Source: CAD feature listing. Evaluate the final solid. Frame: model axes, mm. Give positions to 0.01 mm unless a question says otherwise; leave off trailing zeros. Write each loop counter-clockwise with the first axis right and the second up, starting at its lowest first coordinate (ties: lowest second). Pieces come first, ordered by that corner, then holes. Notation, with made-up numbers: (-40, 45.25) -> (-11, 45.25) arc R24 cw to (-11, 57.25) -> close; hole circle Ø4 at (-27, 60). An arc over 180 degrees is marked (long way). Use one line per item in the form item = value. Start each with the question number.
(1) Cut plane A-A, the plane y = -89. Output: boundary loops of the cut face in (x, z), and give its area (3 significant figures).
(2) Cut plane B-B, the plane x = 65. Output: boundary loops of the cut face in (y, z).
(3) Cut plane C-C, the plane x = 9.5. Output: boundary loops of the cut face in (y, z), and give its area (3 significant figures).
(4) First-contact query: P1, Ø1.5, axis at x = 27.5, z = -1, coming from the -Y side; P2, Ø3, axis at y = -82, z = -4.5, coming from the -X side; P3, Ø1.5, axis at y = -70, z = -2, coming from the -X side; P4, Ø1.5, axis at x = 114, y = -58.5, coming from the +Z side. Flat tips, straight axial feed; report the tip coordinate or a pass-through.
(5) Cut plane D-D, the plane z = -0.85. Count the separate pieces of the cut face and the enclosed holes in it, and give its area (3 significant figures).
(6) Material intervals for line 1 along X through (y, z) = (-136.5, -1.9); line 2 along X through (y, z) = (-113, -2.2); line 3 along X through (y, z) = (-83, -1.7), sorted ascending. Write a range as from..to.
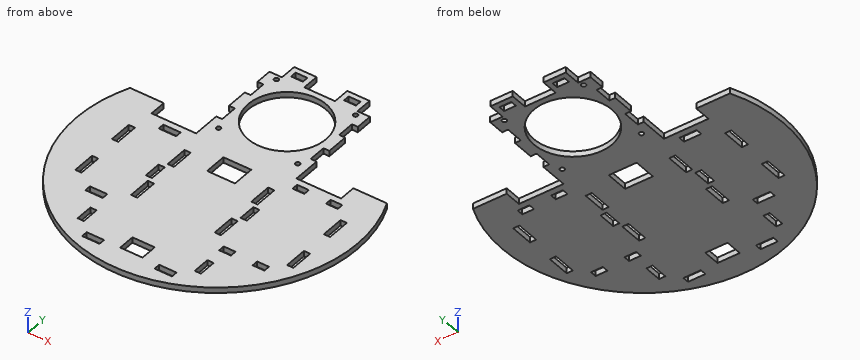
from build123d import *

# Parameters (mm, degrees)
SKETCH1_R           = 35
SKETCH1_R_2         = 2
SKETCH1_W           = 20
SKETCH1_H           = 15
SKETCH1_W_2         = 25
SKETCH1_H_2         = 20
SKETCH1_W_3         = 10.6
SKETCH1_H_3         = 5.6
SKETCH1_W_4         = 15.6
SKETCH1_W_5         = 5.6
SKETCH1_H_4         = 20.6
SKETCH1_H_5         = 15.6
BOSS_EXTRUDE1_DEPTH = 5


with BuildPart() as part:
    # Sketch1 → Boss-Extrude1 (new body)
    with BuildSketch(Plane(origin=(0, 0, 0), x_dir=(-1, 0, 0), z_dir=(0, 0, -1))):
        with BuildLine():
            Line((-25.476672243, 28.966950724), (-36.676672243, 28.966950724))
            Line((-36.676672243, 28.966950724), (-36.676672243, 43.966950724))
            Line((-36.676672243, 43.966950724), (-56.676672243, 43.966950724))
            Line((-56.676672243, 43.966950724), (-56.676672243, 28.966950724))
            Line((-56.676672243, 28.966950724), (-84.276672243, 28.966950724))
            Line((-84.276672243, 28.966950724), (-84.276672243, 43.966950724))
            Line((-84.276672243, 43.966950724), (-104.276672243, 43.966950724))
            Line((-104.276672243, 43.966950724), (-104.276672243, 28.966950724))
            Line((-104.276672243, 28.966950724), (-115.476672243, 28.966950724))
            Line((-115.476672243, 28.966950724), (-115.476672243, 14.266950724))
            Line((-115.476672243, 14.266950724), (-110.176672243, 14.266950724))
            Line((-110.176672243, 14.266950724), (-110.176672243, -1.333049276))
            Line((-110.176672243, -1.333049276), (-115.476672243, -1.333049276))
            Line((-115.476672243, -1.333049276), (-115.476672243, -20.733049276))
            Line((-115.476672243, -20.733049276), (-110.176672243, -20.733049276))
            Line((-110.176672243, -20.733049276), (-110.176672243, -36.333049276))
            Line((-110.176672243, -36.333049276), (-115.476672243, -36.333049276))
            Line((-115.476672243, -36.333049276), (-115.476672243, -61.033049276))
            Line((-115.476672243, -61.033049276), (-155.476672243, -61.033049276))
            Line((-155.476672243, -61.033049276), (-155.476672243, -46.033049276))
            Line((-155.476672243, -46.033049276), (-185.693858461, -46.033049276))
            ThreePointArc((-185.693858461, -46.033049276), (-70.476672243, -223.033049276), (44.740513975, -46.033049276))
            Line((44.740513975, -46.033049276), (14.523327757, -46.033049276))
            Line((14.523327757, -46.033049276), (14.523327757, -61.033049276))
            Line((14.523327757, -61.033049276), (-25.476672243, -61.033049276))
            Line((-25.476672243, -61.033049276), (-25.476672243, -36.333049276))
            Line((-25.476672243, -36.333049276), (-30.776672243, -36.333049276))
            Line((-30.776672243, -36.333049276), (-30.776672243, -20.733049276))
            Line((-30.776672243, -20.733049276), (-25.476672243, -20.733049276))
            Line((-25.476672243, -20.733049276), (-25.476672243, -1.333049276))
            Line((-25.476672243, -1.333049276), (-30.776672243, -1.333049276))
            Line((-30.776672243, -1.333049276), (-30.776672243, 14.266950724))
            Line((-30.776672243, 14.266950724), (-25.476672243, 14.266950724))
            Line((-25.476672243, 14.266950724), (-25.476672243, 28.966950724))
        make_face()
        with Locations((-70.476672243, -11.033049276)):
            Circle(SKETCH1_R, mode=Mode.SUBTRACT)
        with Locations((-34.976672243, 24.466950724)):
            Circle(SKETCH1_R_2, mode=Mode.SUBTRACT)
        with Locations((-105.976672243, 24.466950724)):
            Circle(SKETCH1_R_2, mode=Mode.SUBTRACT)
        with Locations((-105.976672243, -46.533049276)):
            Circle(SKETCH1_R_2, mode=Mode.SUBTRACT)
        with Locations((-34.976672243, -46.533049276)):
            Circle(SKETCH1_R_2, mode=Mode.SUBTRACT)
        with Locations((-70.476672243, -194.533049276)):
            Rectangle(SKETCH1_W, SKETCH1_H, mode=Mode.SUBTRACT)
        with Locations((-70.476672243, -82.033049276)):
            Rectangle(SKETCH1_W_2, SKETCH1_H_2, mode=Mode.SUBTRACT)
        with Locations((-46.676672243, 36.466950724)):
            Rectangle(SKETCH1_W_3, SKETCH1_H_3, mode=Mode.SUBTRACT)
        with Locations((-94.276672243, 36.466950724)):
            Rectangle(SKETCH1_W_3, SKETCH1_H_3, mode=Mode.SUBTRACT)
        with Locations((-7.976672243, -69.533049276)):
            Rectangle(SKETCH1_W_4, SKETCH1_H_3, mode=Mode.SUBTRACT)
        with Locations((17.023327757, -92.033049276)):
            Rectangle(SKETCH1_W_5, SKETCH1_H_4, mode=Mode.SUBTRACT)
        with Locations((-32.976672243, -92.033049276)):
            Rectangle(SKETCH1_W_5, SKETCH1_H_4, mode=Mode.SUBTRACT)
        with Locations((-27.976672243, -114.533049276)):
            Rectangle(SKETCH1_W_5, SKETCH1_H_5, mode=Mode.SUBTRACT)
        with Locations((17.023327757, -137.033049276)):
            Rectangle(SKETCH1_W_5, SKETCH1_H_4, mode=Mode.SUBTRACT)
        with Locations((-7.976672243, -159.533049276)):
            Rectangle(SKETCH1_W_4, SKETCH1_H_3, mode=Mode.SUBTRACT)
        with Locations((-32.976672243, -137.033049276)):
            Rectangle(SKETCH1_W_5, SKETCH1_H_4, mode=Mode.SUBTRACT)
        with Locations((-17.976672243, -184.533049276)):
            Rectangle(SKETCH1_W_5, SKETCH1_H_5, mode=Mode.SUBTRACT)
        with Locations((-37.976672243, -204.533049276)):
            Rectangle(SKETCH1_W_4, SKETCH1_H_3, mode=Mode.SUBTRACT)
        with Locations((-102.976672243, -204.533049276)):
            Rectangle(SKETCH1_W_4, SKETCH1_H_3, mode=Mode.SUBTRACT)
        with Locations((-122.976672243, -184.533049276)):
            Rectangle(SKETCH1_W_5, SKETCH1_H_5, mode=Mode.SUBTRACT)
        with Locations((-125.476672243, -159.533049276)):
            Rectangle(SKETCH1_W_3, SKETCH1_H_3, mode=Mode.SUBTRACT)
        with Locations((-155.476672243, -159.533049276)):
            Rectangle(SKETCH1_W_3, SKETCH1_H_3, mode=Mode.SUBTRACT)
        with Locations((-107.976672243, -137.033049276)):
            Rectangle(SKETCH1_W_5, SKETCH1_H_4, mode=Mode.SUBTRACT)
        with Locations((-172.976672243, -137.033049276)):
            Rectangle(SKETCH1_W_5, SKETCH1_H_4, mode=Mode.SUBTRACT)
        with Locations((-112.976672243, -114.533049276)):
            Rectangle(SKETCH1_W_5, SKETCH1_H_5, mode=Mode.SUBTRACT)
        with Locations((-107.976672243, -92.033049276)):
            Rectangle(SKETCH1_W_5, SKETCH1_H_4, mode=Mode.SUBTRACT)
        with Locations((-172.976672243, -92.033049276)):
            Rectangle(SKETCH1_W_5, SKETCH1_H_4, mode=Mode.SUBTRACT)
        with Locations((-125.476672243, -69.533049276)):
            Rectangle(SKETCH1_W_3, SKETCH1_H_3, mode=Mode.SUBTRACT)
        with Locations((-155.476672243, -69.533049276)):
            Rectangle(SKETCH1_W_3, SKETCH1_H_3, mode=Mode.SUBTRACT)
    extrude(amount=BOSS_EXTRUDE1_DEPTH)


solid = part.part
Geometry says:
q1.outline = (-55.27, -5) -> (-19.82, -5) -> (-19.82, 0) -> (-55.27, 0) -> close; (-14.22, -5) -> (30.18, -5) -> (30.18, 0) -> (-14.22, 0) -> close; (35.78, -5) -> (57.98, -5) -> (57.98, 0) -> (35.78, 0) -> close; (82.98, -5) -> (105.18, -5) -> (105.18, 0) -> (82.98, 0) -> close; (110.78, -5) -> (170.18, -5) -> (170.18, 0) -> (110.78, 0) -> close; (175.78, -5) -> (196.22, -5) -> (196.22, 0) -> (175.78, 0) -> close
q1.area = 1,020 mm^2
q2.outline = (-222.91, -5) -> (-202.03, -5) -> (-202.03, 0) -> (-222.91, 0) -> close; (-187.03, -5) -> (-92.03, -5) -> (-92.03, 0) -> (-187.03, 0) -> close; (-72.03, -5) -> (-45.6, -5) -> (-45.6, 0) -> (-72.03, 0) -> close; (23.54, -5) -> (28.97, -5) -> (28.97, 0) -> (23.54, 0) -> close
q3.outline = (-207.3, -5) -> (-162.33, -5) -> (-162.33, 0) -> (-207.3, 0) -> close; (-156.73, -5) -> (-72.33, -5) -> (-72.33, 0) -> (-156.73, 0) -> close; (-66.73, -5) -> (-61.03, -5) -> (-61.03, 0) -> (-66.73, 0) -> close
q3.area = 675 mm^2
q4.P1 = -215.75
q4.P2 = -54.79
q4.P3 = -52.75
q4.P4 = 0
q5.separate_pieces = 1
q5.enclosed_holes = 29
q5.area = 36,600 mm^2
q6.line_1 = -49.18..-19.82, -14.22..30.18, 35.78..105.18, 110.78..170.18, 175.78..190.14
q6.line_2 = -54.51..25.18, 30.78..110.18, 115.78..195.46
q6.line_3 = -54.74..-19.82, -14.22..30.18, 35.78..57.98, 82.98..105.18, 110.78..170.18, 175.78..195.69
